Design review of the part built by this model. Coordinates are the model's own, in mm. Face numbers are marked on the shaded views. A direction names the side the tool comes from. Give positions to 0.01 mm unless a question says otherwise; leave off trailing zeros. Loops run counter-clockwise (first coordinate to the right, second up) from the corner with the lowest first, then second, coordinate; pieces in that order, holes last.
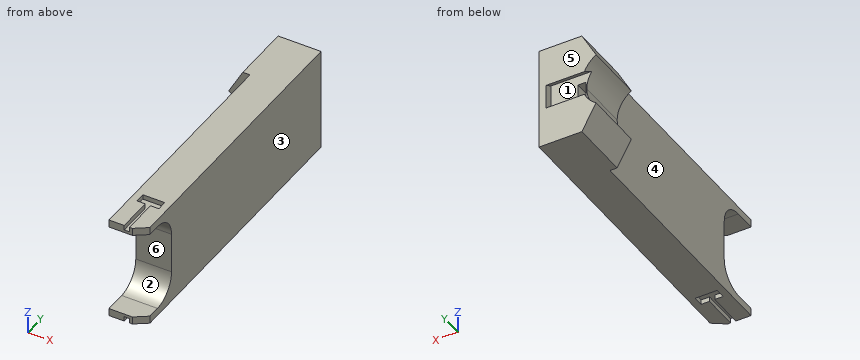
from build123d import *

# Parameters (mm, degrees)
SKETCH2_W               = 18
SKETCH2_H               = 43.5
BOSS_EXTRUDE1_DEPTH     = 25
CUT_EXTRUDE1_DEPTH      = 15
CUT_EXTRUDE1_DEPTH_BACK = 6.951267747
CUT_EXTRUDE2_START      = 0.4
CUT_EXTRUDE2_DEPTH      = 3.3
SKETCH5_W               = 15
SKETCH5_H               = 43.5
BOSS_EXTRUDE2_DEPTH     = 100
SKETCH6_W               = 2.2
SKETCH6_H               = 14.9
CUT_EXTRUDE3_DEPTH      = 2
CUT_EXTRUDE4_START      = -43.5
SKETCH6_3_W             = 2.2
SKETCH6_3_H             = 14.9
CUT_EXTRUDE4_DEPTH      = 2
CUT_EXTRUDE5_DEPTH      = 44.5
SKETCH8_W               = 37.1
SKETCH8_H               = 38
CUT_EXTRUDE6_DEPTH      = 16
FILLET1_R               = 10


with BuildPart() as part:
    # Sketch2 → Boss-Extrude1 (new body)
    with BuildSketch(Plane(origin=(0, 0, 0), x_dir=(1, 0, 0), z_dir=(0, 1, 0))):
        with BuildLine():
            Line((-9, 0), (-9, 21.75))
            Line((-9, 21.75), (-14.951267747, 10.950365309))
            ThreePointArc((-14.951267747, 10.950365309), (-10.583942354, 6.231534486), (-9, 0))
        make_face()
        with BuildLine():
            Line((-9, -21.75), (-9, 0))
            ThreePointArc((-9, 0), (-10.583942354, -6.231534486), (-14.951267747, -10.950365309))
            Line((-14.951267747, -10.950365309), (-9, -21.75))
        make_face()
        Rectangle(SKETCH2_W, SKETCH2_H)
    extrude(amount=BOSS_EXTRUDE1_DEPTH)

    # Sketch3 → Cut-Extrude1 (cut, two sides)
    with BuildSketch(Plane(origin=(-9, 0, 0), x_dir=(0, 0, -1), z_dir=(1, 0, 0))) as cut_extrude1_sk:
        Polygon((-5.15, 25), (5.15, 25), (7.15, 21.535898385), (-7.15, 21.535898385), align=None)
    extrude(amount=CUT_EXTRUDE1_DEPTH, mode=Mode.SUBTRACT)
    extrude(cut_extrude1_sk.sketch, amount=-CUT_EXTRUDE1_DEPTH_BACK, mode=Mode.SUBTRACT)

    # Sketch4 → Cut-Extrude2 (cut)
    with BuildSketch(Plane(origin=(-9, 0, 0), x_dir=(0, 0, -1), z_dir=(1, 0, 0)).offset(CUT_EXTRUDE2_START)):
        with BuildLine():
            Line((3.15, 29.404082691), (3.15, 4.535898385))
            ThreePointArc((3.15, 4.535898385), (0, 1.385898385), (-3.15, 4.535898385))
            Line((-3.15, 4.535898385), (-3.15, 29.404082691))
            ThreePointArc((-3.15, 29.404082691), (0, 32.554082691), (3.15, 29.404082691))
        make_face()
    extrude(amount=CUT_EXTRUDE2_DEPTH, mode=Mode.SUBTRACT)

    # Sketch5 → Boss-Extrude2 (add)
    with BuildSketch(Plane.XZ):
        with Locations((1.5, 0)):
            Rectangle(SKETCH5_W, SKETCH5_H)
    extrude(amount=BOSS_EXTRUDE2_DEPTH)

    # Sketch6 → Cut-Extrude3 (cut)
    with BuildSketch(Plane.XY.offset(21.75)):
        Polygon((-3.1, -85.1), (0.4, -85.1), (2.6, -85.1), (6.1, -85.1), (6.1, -80.9), (-3.1, -80.9), align=None)
        with Locations((1.5, -92.55)):
            Rectangle(SKETCH6_W, SKETCH6_H)
    extrude(amount=-CUT_EXTRUDE3_DEPTH, mode=Mode.SUBTRACT)

    # Sketch6<3> → Cut-Extrude4 (cut)
    with BuildSketch(Plane.XY.offset(21.75).offset(CUT_EXTRUDE4_START)):
        Polygon((-3.1, -85.1), (0.4, -85.1), (2.6, -85.1), (6.1, -85.1), (6.1, -80.9), (-3.1, -80.9), align=None)
        with Locations((1.5, -92.55)):
            Rectangle(SKETCH6_3_W, SKETCH6_3_H)
    extrude(amount=CUT_EXTRUDE4_DEPTH, mode=Mode.SUBTRACT)

    # Sketch7 → Cut-Extrude5 (cut, through all)
    with BuildSketch(Plane.XY.offset(21.75)):
        Polygon((9, -96.358920801), (3.8, -100), (9, -100), align=None)
    extrude(amount=-CUT_EXTRUDE5_DEPTH, mode=Mode.SUBTRACT)

    # Sketch8 → Cut-Extrude6 (cut, through all)
    with BuildSketch(Plane.ZY.offset(6)):
        with Locations((0, -100)):
            Rectangle(SKETCH8_W, SKETCH8_H)
    extrude(amount=-CUT_EXTRUDE6_DEPTH, mode=Mode.SUBTRACT)

    # Fillet1
    fillet1_edges = [part.edges().sort_by_distance(p)[0] for p in [
        (1.5, -81, 18.55),
        (1.5, -81, -18.55),
    ]]
    fillet(fillet1_edges, radius=FILLET1_R)


solid = part.part
Q1. Take a section at C-C (y = -51). Give the boundary of the cut face in (x, z), plus the area to 4 significant figures.
Results:
outline: (-6, -21.75) - (9, -21.75) - (9, 21.75) - (-6, 21.75) - close
area: 652.5 mm2
Q2. Wall thickness on line 1 (X direction, y = -3, z = -13.5); line 2 (Z direction, x = 6, y = -91.5); line 3 (Z direction, x = -6, y = 8): over which ranges is each line inside the solid? List them lowest first.
Results:
line 1: x = -6 to 9
line 2: z = -21.75 to -18.55, 18.55 to 21.75
line 3: z = -21.75 to -3.15, 3.15 to 21.75
Q3. Draft analysis for pull direction Y (two halves, no side actions). For the marked faces 1, 2 and 3, state which applies: pulls with the +Y half, pulls with the -Y half, needs draft (parallel to the pull), parting line crosses it, or undercut.
Results:
face 1: undercut
face 2: pulls with the -Y half
face 3: needs draft
Q4. Take a section at B-B (z = 1.5). Give the boundary of the cut face in (x, y), plus the area to 3 significant figures.
Results:
outline: (-9.09, 0) - (-6, 0) - (-6, -81) - (9, -81) - (9, 25) - (6, 25) - (6, 21.54) - (-5.3, 21.54) - (-5.3, 1.77) - (-8.6, 1.77) - (-8.6, 21.54) - (-9.09, 21.54) - close
area: 1,550 mm2
Q5. Take a section at A-A (x = -1.75). Give the boundary of the cut face in (y, z).
Results:
outline: (-100, -21.75) - (-85.1, -21.75) - (-85.1, -19.75) - (-80.9, -19.75) - (-80.9, -21.75) - (25, -21.75) - (25, -5.15) - (21.54, -7.15) - (21.54, 7.15) - (25, 5.15) - (25, 21.75) - (-80.9, 21.75) - (-80.9, 19.75) - (-85.1, 19.75) - (-85.1, 21.75) - (-100, 21.75) - (-100, 18.55) - (-91, 18.55) arc R10 cw to (-81, 8.55) - (-81, -8.55) arc R10 cw to (-91, -18.55) - (-100, -18.55) - close
Q6. Tool access review of the marked faces 4, 5 and 6: name each direction out of +Z, -Z, +X, -X, +Y, -Y from which nothing blocks a thin tool from reaching the whole face with its end or side.
Results:
face 4: +Z, -Z, -X, -Y
face 5: +Z, -Z, +X, -X, +Y
face 6: +X, -X, -Y
Q7. Insertion check: pin 1 (1 mm diameter, centred on x = 1.5, z = -0.5, fed in from +Y); pin 2 (1 mm diameter, centred on y = -82.5, z = -20.5, fed in from -X); pin 3 (10 mm diameter, centred on x = -8.5, z = -9.5, fed in from -Y). Each pin has a flat end and moves straight along its axis. Give the tip position at first contact, or say it passes through.
Results:
pin 1: stops at y = 21.54
pin 2: stops at x = -6
pin 3: stops at y = -82.51
Q8. Take a section at D-D (z = -12.5). Give the boundary of the cut face in (x, y), plus the area to 3 significant figures.
Results:
outline: (-14.1, 0) - (-6, 0) - (-6, -81.81) - (9, -81.81) - (9, 25) - (-14.1, 25) - close
area: 1,800 mm2
